from build123d import *

# Parameters (mm, degrees)
ESQUISSE1_R        = 18
ESQUISSE1_R_2      = 1.5
BOSS_EXTRU_1_DEPTH = 3


with BuildPart() as part:
    # Esquisse1 → Boss.-Extru.1 (new body)
    with BuildSketch(Plane.XY):
        Circle(ESQUISSE1_R)
        with Locations((5.240453276, 9.386167986)):
            Circle(ESQUISSE1_R_2, mode=Mode.SUBTRACT)
        with Locations((5.508433282, -9.231449657)):
            Circle(ESQUISSE1_R_2, mode=Mode.SUBTRACT)
        with Locations((-10.748886558, -0.154718329)):
            Circle(ESQUISSE1_R_2, mode=Mode.SUBTRACT)
        with BuildLine():
            ThreePointArc((2.485564989, -8.649969172), (4.611711585, -7.728655527), (6.432157603, -6.295025701))
            ThreePointArc((6.432157603, -6.295025701), (7.625396258, -6.875738378), (8.487039823, -7.88500349))
            ThreePointArc((8.487039823, -7.88500349), (9.92431211, -8.79166991), (11.453630047, -8.050736534))
            ThreePointArc((11.453630047, -8.050736534), (13.998549936, 0.201493638), (11.217170127, 8.377057619))
            ThreePointArc((11.217170127, 8.377057619), (9.667160345, 9.073667479), (8.256579008, 8.126009358))
            ThreePointArc((8.256579008, 8.126009358), (7.424340898, 7.092362693), (6.248310551, 6.47754701))
            ThreePointArc((6.248310551, 6.47754701), (4.387356231, 7.858187151), (2.235573373, 8.717924736))
            ThreePointArc((2.235573373, 8.717924736), (2.141865976, 10.041656062), (2.58509342, 11.292493835))
            ThreePointArc((2.58509342, 11.292493835), (2.651653429, 12.990541357), (1.245327334, 13.944502853))
            ThreePointArc((1.245327334, 13.944502853), (-7.173773577, 12.022353042), (-12.86332977, 5.525825479))
            ThreePointArc((-12.86332977, 5.525825479), (-12.691606715, 3.835172702), (-11.165620039, 3.087402491))
            ThreePointArc((-11.165620039, 3.087402491), (-9.854336713, 2.883486477), (-8.73387554, 2.172422163))
            ThreePointArc((-8.73387554, 2.172422163), (-8.999067816, -0.129531624), (-8.667730976, -2.422899035))
            ThreePointArc((-8.667730976, -2.422899035), (-9.767262234, -3.165917684), (-11.072133243, -3.407490345))
            ThreePointArc((-11.072133243, -3.407490345), (-12.575965538, -4.198871447), (-12.698957381, -5.893766319))
            ThreePointArc((-12.698957381, -5.893766319), (-6.824776359, -12.22384668), (1.646159643, -13.902883098))
            ThreePointArc((1.646159643, -13.902883098), (3.02444637, -12.90884018), (2.909041031, -11.213411848))
            ThreePointArc((2.909041031, -11.213411848), (2.429995816, -9.97584917), (2.485564989, -8.649969172))
        make_face(mode=Mode.SUBTRACT)
    extrude(amount=BOSS_EXTRU_1_DEPTH)


solid = part.part
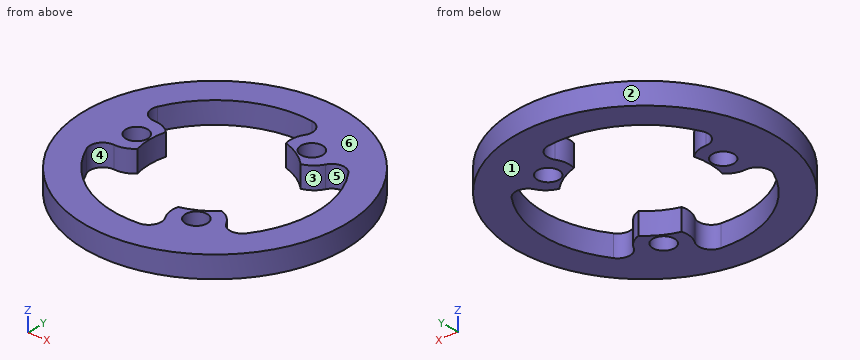
The listing builds one solid part. Answer for the finished solid, in the listing's coordinates (mm). Face numbers are marked on the shaded views. A direction names the side the tool comes from. Round coordinates to 2 decimals unless told otherwise and drop trailing zeros. Write each loop counter-clockwise with the first axis right and the second up, starting at its lowest first coordinate (ties: lowest second). Pieces come first, ordered by that corner, then holes. Notation, with made-up numbers: M 88,-32.75 L 128,-32.75 A17 ccw 128,-2.75 Z; hole C 85,35.5 d3. An arc over 180 degrees is marked long. Write each question's results on one line, items separated by ' | '. Start each with the question number.
Item 1: Find section B-B on z = 0.45. Give the number of separate pieces and of enclosed holes in the cut face, and give its area (3 significant figures).
Item 2: Which of the six approach directions +Z, -Z, +X, -X, +Y, -Y give full straight-line access (tool end or side, diameter ignored) to the marked faces 5 and 6?
Item 3: Find section A-A on x = 0. Write down the section's boundary in (y, z), and give its area (3 significant figures).
Item 4: Find section D-D on x = -14. Write down the section's boundary in (y, z), and give its area (3 significant figures).
Item 5: Straight lines are drawn through the part: probe 1 along X at (y, z) = (-7.5, 2); probe 2 along Y at (x, z) = (-12, 2.05); probe 3 along X at (y, z) = (-10.5, 1.95). For each, find the intervals that lie inside material, in ascending order.
Item 6: The mould has two halves that part along Y. Classify the marked faces 1, 2, 3 and 4: +Y half, -Y half, draft (parallel to the pull), parting line (faces both ways), or undercut.
Item 7: Find section C-C on x = -4.5. Write down the section's boundary in (y, z), and give its area (3 significant figures).
Item 8: Given pin 1 Ø1 at (x, z) = (1, 1.5) entering from +Y, flat-ended and moving along its own axis, determine where the tip first touches the part or whether it passes through.
Answer block:
1) separate pieces: 1 | enclosed holes: 4 | area: 484 mm²
2) face 5: +Z, -Z | face 6: +Z, +X, -X, +Y, -Y
3) outline: M -18,0 L -14,0 L -14,3 L -18,3 Z; M 14,0 L 18,0 L 18,3 L 14,3 Z | area: 24.0 mm²
4) outline: M -11.31,0 L 11.31,0 L 11.31,3 L -11.31,3 Z | area: 67.9 mm²
5) probe 1: x = -16.36 to -11.82, 4.97 to 8.24, 11.82 to 16.36 | probe 2: y = -13.42 to -7.21, -3.65 to -0.98, 0.67 to 3.25, 7.21 to 13.42 | probe 3: x = -14.62 to -9.26, 2.56 to 4.71, 6.31 to 14.62
6) face 1: draft | face 2: parting line | face 3: undercut | face 4: undercut
7) outline: M -17.43,0 L -13.26,0 L -13.26,3 L -17.43,3 Z; M 13.26,0 L 17.43,0 L 17.43,3 L 13.26,3 Z | area: 25.0 mm²
8) pin 1: stops at y = 17.99
